Answer from the drawing. Dimensions are ordinates in mm from the lowest x, y and z of the part. Coordinates: 2 decimals unless noted, no trailing zeros. Order: outer loops, then holes, each group sorted by start corner. A loop starts at its lowest first (then second) coordinate and runs counter-clockwise, first axis right, second up. Notation, with made-up numbers: (60, 62) -> (77, 62) arc R24 ccw to (77, 85) -> close; hole circle Ø1 at (41, -35). An arc over 180 degrees is marked (long way). Answer in a Markdown table with one row per item.
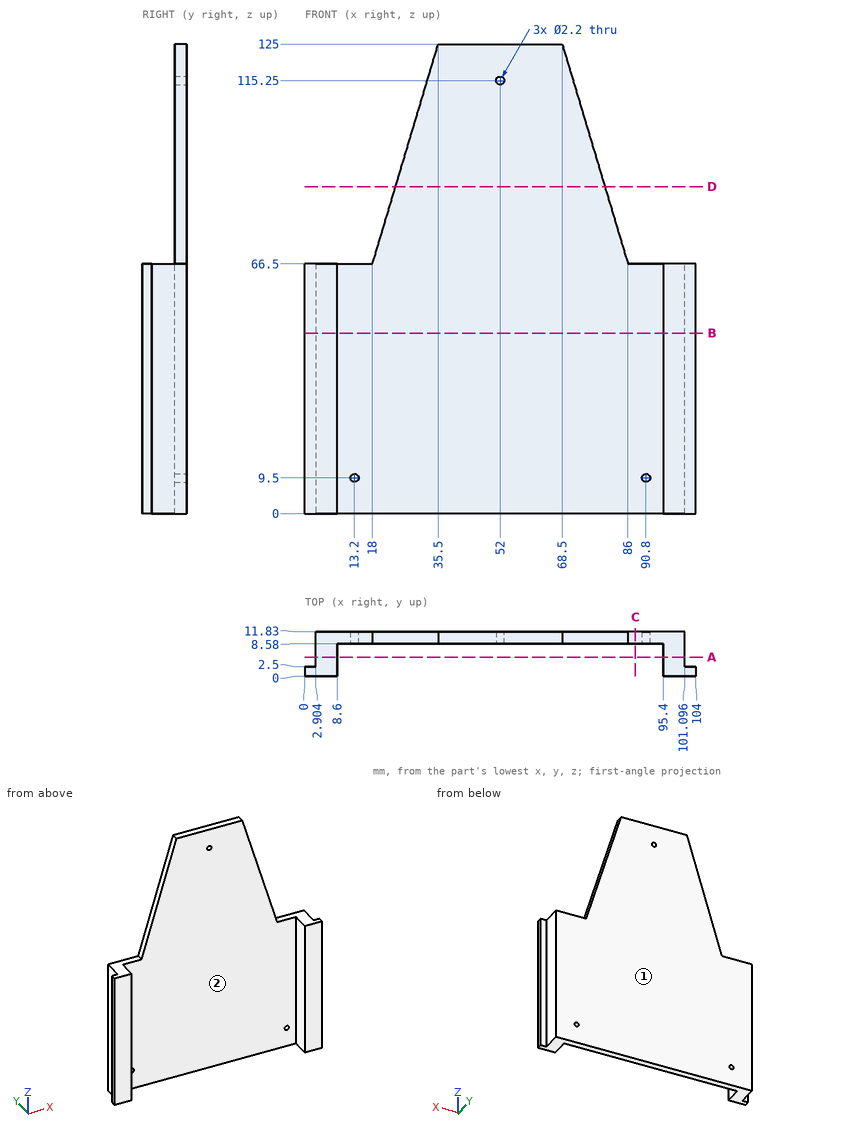
Q1. The part is cut by section B-B (z = 48). Write down the section's boundary in (x, y).
Outcome:
| item | result |
|---|---|
| outline | (0, 0) -> (8.6, 0) -> (8.6, 8.58) -> (95.4, 8.58) -> (95.4, 0) -> (104, 0) -> (104, 2.5) -> (101.1, 2.5) -> (101.1, 11.83) -> (2.9, 11.83) -> (2.9, 2.5) -> (0, 2.5) -> close |
Q2. Given pin 1 (4 mm diameter, centred on y = 6, z = 54, fed in from -X); pin 2 (3 mm diameter, centred on x = 43.5, z = 47.5, fed in from -Y); pin 3 (3 mm diameter, centred on x = 103, z = 21, fed in from +Y), each flat-ended and moving along its own axis, determine where each tip first touches the part or whether it passes through.
Outcome:
| item | result |
|---|---|
| pin 1 | x = 2.9 |
| pin 2 | y = 8.58 |
| pin 3 | y = 2.5 |
Q3. For a pull along X with two mould halves and no side action, classify the marked faces 1 and 2 as pulls with the +X half, pulls with the -X half, needs draft (parallel to the pull), parting line crosses it, or undercut.
Outcome:
| item | result |
|---|---|
| face 1 | needs draft |
| face 2 | undercut |
Q4. The part is cut by section A-A (y = 5). Write down the section's boundary in (x, z).
Outcome:
| item | result |
|---|---|
| outline | (2.9, 0) -> (8.6, 0) -> (8.6, 66.5) -> (2.9, 66.5) -> close; (95.4, 0) -> (101.1, 0) -> (101.1, 66.5) -> (95.4, 66.5) -> close |
Q5. Consider line 1 (Z direction, x = 13.2, y = 10.2); line 2 (X direction, y = 1.25, z = 16); line 3 (X direction, y = 7.25, z = 64.5). Determine where each line is inside the solid, lowest interval first.
Outcome:
| item | result |
|---|---|
| line 1 | 0 to 8.4, 10.6 to 66.5 |
| line 2 | 0 to 8.6, 95.4 to 104 |
| line 3 | 2.9 to 8.6, 95.4 to 101.1 |
Q6. The part is cut by section C-C (x = 88). Write down the section's boundary in (y, z), then the cut area to 3 significant figures.
Outcome:
| item | result |
|---|---|
| outline | (8.58, 0) -> (11.83, 0) -> (11.83, 66.5) -> (8.58, 66.5) -> close |
| area | 216 mm² |
Q7. The part is cut by section D-D (z = 87). Write down the section's boundary in (x, y).
Outcome:
| item | result |
|---|---|
| outline | (24.13, 8.58) -> (79.87, 8.58) -> (79.87, 11.83) -> (24.13, 11.83) -> close |
